Work out the finished part from the listing and answer in its coordinate system (mm). A direction names the side the tool comes from. Coordinates: 2 decimals unless noted, no trailing zeros. Order: outer loops, then holes, each group sorted by start corner. A loop starts at its lowest first (then second) coordinate and runs counter-clockwise, first axis right, second up.
```python
from build123d import *

# Parameters (mm, degrees)
IZIM1_R                     = 5.04
Y_KSEKLIK_EKSTR_ZYON1_DEPTH = 10.35
PAH1_SIZE                   = 0.68
IZIM2_R                     = 4.26
KES_EKSTR_ZYON1_DEPTH       = 10.35
Y_KSEKLIK_EKSTR_ZYON2_DEPTH = 9.67
KES_EKSTR_ZYON2_DEPTH       = 16.20471315
KES_EKSTR_ZYON2_DEPTH_BACK  = 16.20471315
KES_EKSTR_ZYON3_DEPTH       = 16.20471315
KES_EKSTR_ZYON3_DEPTH_BACK  = 16.20471315
RADYUS1_R                   = 0.84
RADYUS4_R                   = 0.84
RADYUS5_R                   = 1.57
RADYUS6_R                   = 1.57


with BuildPart() as part:
    # Çizim1 → Yükseklik-Ekstrüzyon1 (new body)
    with BuildSketch(Plane.XY):
        Circle(IZIM1_R)
    extrude(amount=Y_KSEKLIK_EKSTR_ZYON1_DEPTH)

    # Pah1
    pah1_edges = [part.edges().sort_by_distance(p)[0] for p in [
        (-5.04, 0, 0),
    ]]
    chamfer(pah1_edges, length=PAH1_SIZE)

    # Çizim2 → Kes-Ekstrüzyon1 (cut)
    with BuildSketch(Plane.XY.offset(10.35)):
        Circle(IZIM2_R)
    extrude(amount=-KES_EKSTR_ZYON1_DEPTH, mode=Mode.SUBTRACT)

    # Çizim3 → Yükseklik-Ekstrüzyon2 (add)
    with BuildSketch(Plane.XY.offset(10.35)):
        Polygon((5.01, 0.44), (9.92, 0.85), (9.92, 0), (9.92, -0.85), (5.01, -0.44), (5.01, 0), align=None)
        Polygon((-5.01, 0), (-5.01, 0.44), (-9.92, 0.85), (-9.92, 0), (-9.92, -0.85), (-5.01, -0.44), align=None)
    extrude(amount=-Y_KSEKLIK_EKSTR_ZYON2_DEPTH)

    # Çizim4 → Kes-Ekstrüzyon2 (cut, two sides: drawn at the far end of the back side and taken through both)
    with BuildSketch(Plane(origin=(0.001795297, -0.021499782, 0), x_dir=(-0.9965317468742466, -0.08321344525833854, 0), z_dir=(0.08321344525833854, -0.9965317468742466, 0)).offset(-KES_EKSTR_ZYON2_DEPTH_BACK)):
        Polygon((9.956326357, -0.68), (5.879953823, -0.68), (9.956326357, -4.05), align=None)
    extrude(amount=KES_EKSTR_ZYON2_DEPTH + KES_EKSTR_ZYON2_DEPTH_BACK, mode=Mode.SUBTRACT)

    # Çizim5 → Kes-Ekstrüzyon3 (cut, two sides: drawn at the far end of the back side and taken through both)
    with BuildSketch(Plane(origin=(-0.001795297, -0.021499782, 0), x_dir=(-0.9965317468742466, 0.08321344525833854, 0), z_dir=(-0.08321344525833854, -0.9965317468742466, 0)).offset(-KES_EKSTR_ZYON3_DEPTH_BACK)):
        Polygon((-9.956326357, -4.05), (-5.879953823, -0.68), (-9.956326357, -0.68), align=None)
    extrude(amount=KES_EKSTR_ZYON3_DEPTH + KES_EKSTR_ZYON3_DEPTH_BACK, mode=Mode.SUBTRACT)

    # Radyus1
    radyus1_edges = [part.edges().sort_by_distance(p)[0] for p in [
        (5.900717461, 0.003586632, 0.68),
    ]]
    fillet(radyus1_edges, radius=RADYUS1_R)

    # Radyus4
    radyus4_edges = [part.edges().sort_by_distance(p)[0] for p in [
        (-5.900717461, 0.003586632, 0.68),
    ]]
    fillet(radyus4_edges, radius=RADYUS4_R)

    # Radyus5
    radyus5_edges = [part.edges().sort_by_distance(p)[0] for p in [
        (-9.92, 0, 10.35),
    ]]
    fillet(radyus5_edges, radius=RADYUS5_R)

    # Radyus6
    radyus6_edges = [part.edges().sort_by_distance(p)[0] for p in [
        (9.92, 0, 10.35),
    ]]
    fillet(radyus6_edges, radius=RADYUS6_R)


solid = part.part
```
1. The part is cut by section D-D (x = -7.75). Determine the outline of the cut face in (y, z), plus the area to 3 significant figures.
2. The part is cut by section A-A (x = 0). Determine the outline of the cut face in (y, z), plus the area to 3 significant figures.
3. For faces 5 (the flat face through (-7.436, 0.643, 5.583)), 6 (the flat face through (-7.505, -0.648, 5.583)), 7 (the cylindrical face through (-9.47, -0.01, 9.88)), determine the directions among +Z, -Z, +X, -X, +Y, -Y from which every point of the face is accessible in a straight line to the end or side of a thin tool.
4. The part is cut by section C-C (z = 3.5). Determine the outline of the cut face in (x, y).
5. Flat-ended cylindrical pins translate along their axes: pin 1 (5 mm diameter, centred on x = -5, z = 5, fed in from +Y); pin 2 (1 mm diameter, centred on y = -0.5, z = 2.5, fed in from +X). Find the tip coordinate at first contact, or state that the pin passes through.
6. Consider probe 1 along Y at (x, z) = (0, 7.25); probe 2 along Y at (x, z) = (-1.5, 8.25); probe 3 along X at (y, z) = (3.75, 5.5). Determine where each line is inside the solid, lowest interval first.
7. The part is cut by section B-B (z = 6.5). Determine the outline of the cut face in (x, y), plus the area to 3 significant figures.
8. The mould has two halves that part along Y. Classify faces 1 (the cylindrical face through (0.1, 5.04, 5.45)), 2 (the flat face through (4, -2, 10.35)), 3 (the cylindrical face through (-0.92, -4.16, 5.25)), 4 (the flat face through (8.088, -0.024, 2.484)): released by +Y, released by -Y, zero draft, split by the parting line, or undercut.
Worked out:
1. outline: (-0.67, 2.25) - (0.67, 2.16) - (0.67, 10.35) - (-0.67, 10.35) - close
1. area: 10.9 mm2
2. outline: (-5.04, 0.68) - (-4.36, 0) - (-4.26, 0) - (-4.26, 10.35) - (-5.04, 10.35) - close; (4.26, 0) - (4.36, 0) - (5.04, 0.68) - (5.04, 10.35) - (4.26, 10.35) - close
2. area: 15.7 mm2
3. face 5: +Z, -Z, +Y
3. face 6: +Z, -Z, -Y
3. face 7: +Z, -X, +Y, -Y
4. outline: (-9.39, 0.81) - (-9.26, -0.79) - (-5.02, -0.44) arc R5.04 ccw to (5.02, -0.44) - (9.26, -0.79) - (9.39, 0.81) - (5.02, 0.44) arc R5.04 ccw to (-5.02, 0.44) - close; hole circle Ø8.52 at (0, 0)
5. pin 1: stops at y = 4.38
5. pin 2: stops at x = 8.68
6. probe 1: y = -5.04 to -4.26, 4.26 to 5.04
6. probe 2: y = -4.81 to -3.99, 3.99 to 4.81
6. probe 3: x = -3.37 to -2.02, 2.02 to 3.37
7. outline: (-9.92, -0.85) - (-5.02, -0.44) arc R5.04 ccw to (5.02, -0.44) - (9.92, -0.85) - (9.92, 0.85) - (5.02, 0.44) arc R5.04 ccw to (-5.02, 0.44) - (-9.92, 0.85) - close; hole circle Ø8.52 at (0, 0)
7. area: 35.4 mm2
8. face 1: released by +Y
8. face 2: zero draft
8. face 3: undercut
8. face 4: released by -Y
